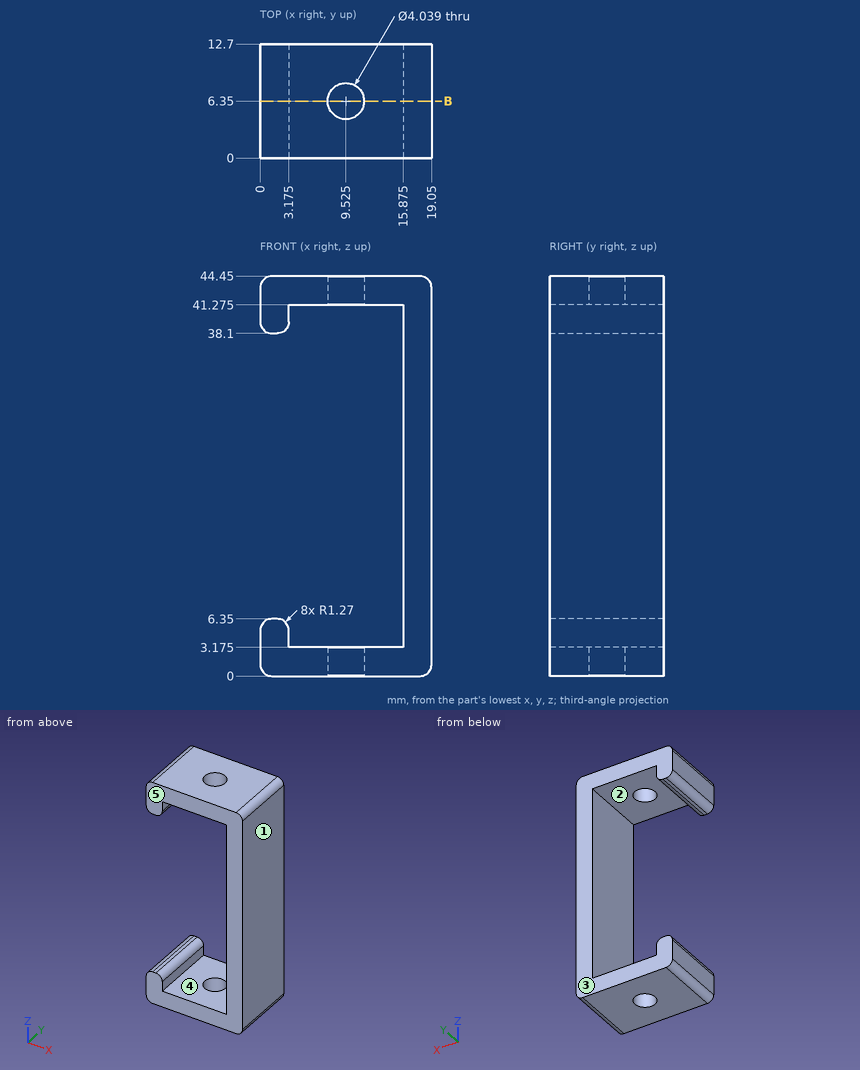
The drawing under review shows one solid part. Ordinate dimensions are in mm from its lowest x, y, z. A direction names the side the tool comes from. Coordinates: 2 decimals unless noted, no trailing zeros. Use CSV: the item, a comma, the result in double quotes. Start each with the question number.
Item 1: Draft analysis for pull direction X (two halves, no side actions). For the marked faces 1, 2 and 3, state which applies: pulls with the +X half, pulls with the -X half, needs draft (parallel to the pull), parting line crosses it, or undercut.
Item 2: For the marked faces 4 and 5, list the 3-axis set-ups (+Z, -Z, +X, -X, +Y, -Y) from which the entire face can be reached by the end or side of a thin tool; tool diameter is ignored.
Item 3: Insertion check: pin 1 (4 mm diameter, centred on y = 5.5, z = 25.5, fed in from -X) (3 decimals). The pin has a flat end and moves straight along its axis. Give the tip position at first contact, or say it passes through.
Item 4: Wall thickness on probe 1 along Z at (x, y) = (1, 3.75): over which ranges is the line inside the solid? List them lowest first.
Item 5: We need section B-B, the plane y = 6.35. Give the number of separate pieces and of enclosed holes in the cut face, then the cut area to 3 significant figures.
Derived:
1,face 1,"pulls with the +X half"
1,face 2,"undercut"
1,face 3,"needs draft"
2,face 4,"+Y, -Y"
2,face 5,"+Z, -Z, +X, -X, -Y"
3,pin 1,"stops at x = 15.875"
4,probe 1,"z = 0.03 to 6.32, 38.13 to 44.42"
5,separate pieces,"3"
5,enclosed holes,"0"
5,area,"234 mm^2"
